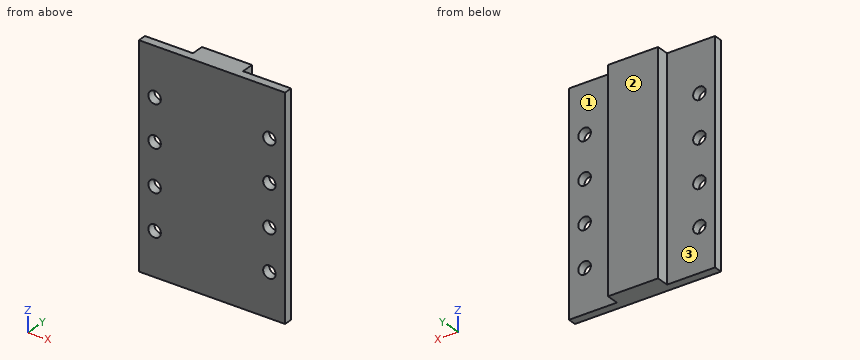
from build123d import *

# Parameters (mm, degrees)
SKETCH_1_W                  = 35
SKETCH_1_H                  = 52
EXTRUDE_1_DEPTH             = 2
EXTRUDE_2_REACH             = 33.405
SKETCH_2_W                  = 12
SKETCH_2_H                  = 3
EXTRUDE_2_DIRECTION_2_REACH = 33.405
SKETCH_3_R                  = 1.5
CUT_EXTRUDE_1_DEPTH         = 10


with BuildPart() as part:
    # Эскиз1 → Бобышка-Вытянуть1 (new body)
    with BuildSketch(Plane(origin=(0, 0, 0), x_dir=(1, 0, 0), z_dir=(0, 1, 0))):
        Rectangle(SKETCH_1_W, SKETCH_1_H)
    extrude(amount=EXTRUDE_1_DEPTH)

    # Бобышка-Вытянуть2: up to this face of the body (flat: up to its plane)
    extrude_2_end = Plane(part.part.faces().sort_by_distance((0, 1, 26))[0])
    # Эскиз2 → Бобышка-Вытянуть2 (add, up to the picked face)
    with BuildSketch(Plane.XY, mode=Mode.PRIVATE) as extrude_2_sk1:
        with Locations((0, 3.5)):
            Rectangle(SKETCH_2_W, SKETCH_2_H)
    extrude_2_tool1 = split(extrude(extrude_2_sk1.sketch, amount=EXTRUDE_2_REACH, mode=Mode.PRIVATE), bisect_by=extrude_2_end, keep=Keep.BOTH, mode=Mode.PRIVATE)
    add(extrude_2_tool1.solids().sort_by(Axis((0, 3.5, 0), (0, 0, 1)))[0])

    # Бобышка-Вытянуть2 direction 2: up to this face of the body (flat: up to its plane)
    extrude_2_direction_2_end = Plane(part.part.faces().sort_by_distance((0, 1, -26))[0])
    # Эскиз2 → Бобышка-Вытянуть2 direction 2 (add, up to the picked face)
    with BuildSketch(Plane.XY, mode=Mode.PRIVATE) as extrude_2_direction_2_sk1:
        with Locations((0, 3.5)):
            Rectangle(SKETCH_2_W, SKETCH_2_H)
    extrude_2_direction_2_tool1 = split(extrude(extrude_2_direction_2_sk1.sketch, amount=-EXTRUDE_2_DIRECTION_2_REACH, mode=Mode.PRIVATE), bisect_by=extrude_2_direction_2_end, keep=Keep.BOTH, mode=Mode.PRIVATE)
    add(extrude_2_direction_2_tool1.solids().sort_by(Axis((0, 3.5, 0), (0, 0, -1)))[0])

    # Эскиз3 → Вырез-Вытянуть1 (cut)
    with BuildSketch(Plane(origin=(0, 2, 0), x_dir=(1, 0, 0), z_dir=(0, 1, 0))):
        with Locations(Location((13.75, 15.6, 0), (0, 0, 270))):
            Circle(SKETCH_3_R)
        with Locations(Location((-13.75, 15.6, 0), (0, 0, 270))):
            Circle(SKETCH_3_R)
        with Locations(Location((-13.75, 5.6, 0), (0, 0, 270))):
            Circle(SKETCH_3_R)
        with Locations(Location((13.75, 5.6, 0), (0, 0, 270))):
            Circle(SKETCH_3_R)
        with Locations(Location((-13.75, -4.4, 0), (0, 0, 270))):
            Circle(SKETCH_3_R)
        with Locations(Location((13.75, -4.4, 0), (0, 0, 270))):
            Circle(SKETCH_3_R)
        with Locations(Location((-13.75, -14.4, 0), (0, 0, 270))):
            Circle(SKETCH_3_R)
        with Locations(Location((13.75, -14.4, 0), (0, 0, 270))):
            Circle(SKETCH_3_R)
    extrude(amount=-CUT_EXTRUDE_1_DEPTH, mode=Mode.SUBTRACT)


solid = part.part
CAD build for the part. Positions are in the model's coordinates, mm. Face numbers are marked on the shaded views. A direction names the side the tool comes from. Round coordinates to 2 decimals unless told otherwise and drop trailing zeros. Write each loop counter-clockwise with the first axis right and the second up, starting at its lowest first coordinate (ties: lowest second). Pieces come first, ordered by that corner, then holes. Notation, with made-up numbers: (41, -4.75) -> (77, -4.75) arc R11 cw to (77, 0.25) -> close; hole circle Ø3 at (71, 85.5). An arc over 180 degrees is marked (long way). Answer as a JSON object with one key per item and string values.
(1) Band-saw the part on D-D, the plane y = 4.4. List the corners of the cut face in (x, z).
Reported:
{"outline": "(-6, -26) -> (6, -26) -> (6, 26) -> (-6, 26) -> close"}
(2) Band-saw the part on A-A, the plane z = -5.6. List the corners of the cut face in (x, y), then the cut area to 3 significant figures.
Reported:
{"outline": "(-17.5, 0) -> (-15.25, 0) -> (-15.25, 2) -> (-17.5, 2) -> close; (-12.25, 0) -> (12.25, 0) -> (12.25, 2) -> (6, 2) -> (6, 5) -> (-6, 5) -> (-6, 2) -> (-12.25, 2) -> close; (15.25, 0) -> (17.5, 0) -> (17.5, 2) -> (15.25, 2) -> close", "area": "94.0 mm^2"}
(3) Pin check, flat tips, straight feed: P1, Ø5, axis at x = 13.75, z = 4.4, coming from the +Y side; P2, Ø0.9, axis at y = 3, z = 3, coming from the +X side; P3, Ø0.9, axis at y = 4, z = 5, coming from the -X side. Stop position of each tip, or through.
Reported:
{"P1": "stops at y = 2", "P2": "stops at x = 6", "P3": "stops at x = -6"}
(4) Which spindle directions (+Z, -Z, +X, -X, +Y, -Y) get a long thin tool onto all of the face, cutting with end or side? Do the marked faces 1, 2 and 3. Say none if no direction does.
Reported:
{"face 1": "+Z, -Z, +X, +Y", "face 2": "+Z, -Z, +X, -X, +Y", "face 3": "+Z, -Z, -X, +Y"}
(5) Band-saw the part on B-B, the plane x = -13.75. List the corners of the cut face in (y, z).
Reported:
{"outline": "(0, -26) -> (2, -26) -> (2, -17.1) -> (0, -17.1) -> close; (0, -14.1) -> (2, -14.1) -> (2, -7.1) -> (0, -7.1) -> close; (0, -4.1) -> (2, -4.1) -> (2, 2.9) -> (0, 2.9) -> close; (0, 5.9) -> (2, 5.9) -> (2, 12.9) -> (0, 12.9) -> close; (0, 15.9) -> (2, 15.9) -> (2, 26) -> (0, 26) -> close"}
(6) Probe probe 1 along X at (y, z) = (1.5, 14.4); probe 2 along Y at (x, z) = (-13, -2); probe 3 along X at (y, z) = (4.6, 9). List the from-to ranges inside material, lowest first. Write a range as [from, to].
Reported:
{"probe 1": "x = [-17.5, -15.25], [-12.25, 12.25], [15.25, 17.5]", "probe 2": "y = [0, 2]", "probe 3": "x = [-6, 6]"}
(7) Band-saw the part on C-C, the plane y = 1.2. Count the separate pieces of the cut face and the enclosed holes in it, then the cut area to 3 significant figures.
Reported:
{"separate pieces": "1", "enclosed holes": "8", "area": "1,760 mm^2"}
